The listing builds one solid part. Answer for the finished solid, in the listing's coordinates (mm). Face numbers are marked on the shaded views. A direction names the side the tool comes from. Give positions to 0.01 mm unless a question says otherwise; leave off trailing zeros. Order: outer loops, then holes, each group sorted by start corner. A loop starts at its lowest first (then second) coordinate and runs counter-clockwise, first axis right, second up. Notation, with made-up numbers: (-28.5, 6.25) -> (-22.5, 6.25) arc R5 cw to (-22.5, 12.25) -> close; hole circle Ø11 at (41, 18). An arc over 180 degrees is marked (long way). Answer as a JSON object with one key per item and string values. Group by question number.
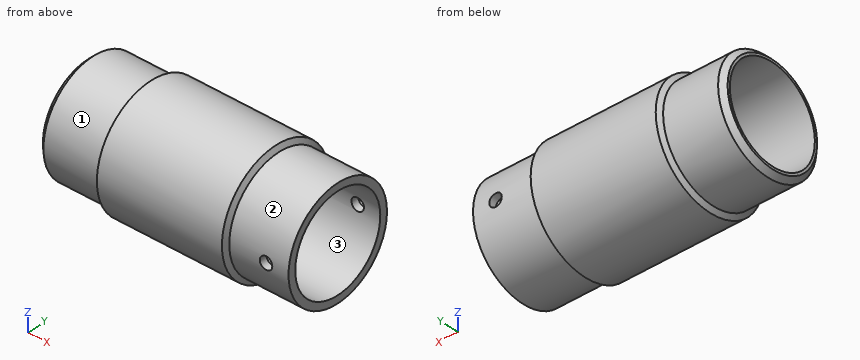
Autodesk Inventor part; units mm, degrees
ref_plane "YZ Plane" through (0, 0, 0) normal (1, 0, 0) x (0, 1, 0)
ref_plane "XZ Plane" through (0, 0, 0) normal (0, 1, 0) x (-1, 0, 0)
ref_plane "XY Plane" through (0, 0, 0) normal (0, 0, 1) x (1, 0, 0)
sketch "Profile" plane through (0, 0, 0) normal (0, 0, 1) x (1, 0, 0)
  line L0 (-12, 0) -> (-12, 11)
  line L1 (-12, 11) -> (0, 11)
  line L2 (0, 11) -> (0.5774, 12)
  line L3 (0.5774, 12) -> (25.5774, 12)
  line L4 (25.5774, 12) -> (26.1547, 11)
  line L5 (26.1547, 11) -> (38, 11)
  line L6 (38, 11) -> (38, 0)
  line L7 (-12, 0) -> (0, 0)
  line L8 (0, 0) -> (0, 9)
  line L9 (0, 9) -> (30, 9)
  line L10 (30, 9) -> (30, 0)
  line L11 (30, 0) -> (38, 0)
  line L12 (-22, 0) -> (48, 0) construction
  line L13 (0, 11) -> (0, 9) construction
  dimension "BodyLength" = 50
  dimension "d1" = 11
  dimension "d3" = 120
  dimension "d4" = 120
  dimension "d5" = 25
  dimension "d6" = 12
  dimension "d16" = 8
  dimension "d29" = 1
  dimension "d30" = 9
revolve "ProfileRevolveFeature" add sketch "Profile" angle 360 about axis through (-10, 0, 0) along (1, 0, 0)
sketch "InsideHole" plane through (-12, 0, 0) normal (-1, 0, 0) x (0, 0, 1)
  circle A0 centre (0, 0) radius 9 construction
hole "InsideHoleFeature" at (-12, 0, 0) direction (1, 0, 0) diameter 19 end through all
chamfer "EndChamferFeature" distance 1 angle 45 1 edges at (-12, -11, 0)
sketch "CapMountHole" plane through (0, 0, 0) normal (0, 1, 0) x (-1, 0, 0)
  line L0 (-38, 11) -> (-38, -11) construction
  line L1 (15.2, 0) -> (-91.2, 0) construction
  circle A0 centre (-33.5, 0) radius 1.25
  point P0 (0, 0)
  dimension "d31" = 4.5
  dimension "d39" = 2.5
extrude "CapMountHoleFeature" cut sketch "CapMountHole" along normal through all both and the other way through all
equation "\"d5\" = 0.5 * BodyLength"
equation "\"d6\" = 0.24 * BodyLength"
properties part number "BackPair1PistonBody"
(1) A cutting plane is placed at D-D (x = -3.5). Determine the outline of the cut face in (y, z), and give its area (3 significant figures).
(2) Which of the six approach directions +Z, -Z, +X, -X, +Y, -Y give full straight-line access (tool end or side, diameter ignored) to the marked faces 1, 2 and 3?
(3) Flat-ended cylindrical pins translate along their axes: pin 1 Ø2 at (x, z) = (31, -5.5) entering from -Y; pin 2 Ø4 at (x, z) = (4, -4.5) entering from +Y; pin 3 Ø2 at (x, z) = (33.5, 0) entering from -Y; pin 4 Ø3 at (x, z) = (33.5, 0) entering from +Y. Find the tip coordinate at first contact, or state that the pin passes through.
(4) A cutting plane is placed at A-A (y = 0). Determine the outline of the cut face in (x, z).
(5) A cutting plane is placed at B-B (x = 7). Determine the outline of the cut face in (y, z), and give its area (3 significant figures).
(6) Find the intervals of material crossed by line 1 along Z through (x, y) = (30, 0.25); line 2 along Z through (x, y) = (13, 0); line 3 along X through (y, z) = (-9.95, 0), in increasing order. Write a range as [from, to].
(7) A cutting plane is placed at C-C (x = 33). Determine the outline of the cut face in (y, z).
Check sheet entries:
{
 "1": {"outline": "circle Ø22 at (0, 0); hole circle Ø19 at (0, 0)", "area": "96.6 mm2"},
 "2": {"face 1": "-X", "face 2": "+X", "face 3": "+X, -X"},
 "3": {"pin 1": "stops at y = -10.04", "pin 2": "stops at y = 11.74", "pin 3": "passes through", "pin 4": "stops at y = 11"},
 "4": {"outline": "(-12, -10) -> (-11, -11) -> (0, -11) -> (0.58, -12) -> (25.58, -12) -> (26.15, -11) -> (38, -11) -> (38, -9.5) -> (-12, -9.5) -> close; (-12, 9.5) -> (38, 9.5) -> (38, 11) -> (26.15, 11) -> (25.58, 12) -> (0.58, 12) -> (0, 11) -> (-11, 11) -> (-12, 10) -> close"},
 "5": {"outline": "circle Ø24 at (0, 0); hole circle Ø19 at (0, 0)", "area": "169 mm2"},
 "6": {"line 1": "z = [-11, -9.5], [9.5, 11]", "line 2": "z = [-12, -9.5], [9.5, 12]", "line 3": "x = [-12, 32.25], [34.75, 38]"},
 "7": {"outline": "(-10.94, -1.15) arc R11 ccw to (10.94, -1.15) -> (9.43, -1.15) arc R9.5 cw to (-9.43, -1.15) -> close; (-10.94, 1.15) -> (-9.43, 1.15) arc R9.5 cw to (9.43, 1.15) -> (10.94, 1.15) arc R11 ccw to start"}
}
